For this review, take the finished solid that the model builds, in its own axes (mm). Give positions to 0.01 mm unless a question says otherwise; leave off trailing zeros. Order: outer loops, then holes, each group sorted by start corner. A loop starts at its lowest first (then second) coordinate and runs counter-clockwise, first axis right, second up.
Item 1: For probe 1 along X at (y, z) = (0.3, 96); probe 2 along Y at (x, z) = (0.2, 120); probe 3 along Y at (x, z) = (-0.4, 152), list the stretches that pass through material, from the lowest coordinate up.
Item 2: Consider section A-A (z = 177.5). Give the boundary of the cut face in (x, y).
Item 3: For P1, Ø2, axis at x = -0.5, z = 110, coming from the +Y side; P2, Ø1, axis at x = 1.5, y = 4, coming from the +Z side; P3, Ø1.5, axis at y = 1.5, z = 239.5, coming from the +X side, all flat-tipped, find the tip position at first contact; note any pin that passes through.
Autodesk Inventor part; units mm, degrees
ref_plane "YZ Plane" through (0, 0, 0) normal (1, 0, 0) x (0, 1, 0)
ref_plane "XZ Plane" through (0, 0, 0) normal (0, 1, 0) x (-1, 0, 0)
ref_plane "XY Plane" through (0, 0, 0) normal (0, 0, 1) x (1, 0, 0)
sketch "Szkic1" plane through (0, 0, 0) normal (0, 0, 1) x (1, 0, 0)
  circle A0 centre (0, 0) radius 1
  dimension "d0" = 2
sketch "Szkic4" plane through (0, 0, 0) normal (1, 0, 0) x (0, 1, 0)
  line L0 (0, 0) -> (0, 263.8767)
  arc A0 (1.817, 265.8683) -> (0, 263.8767) centre (2, 263.8767) ccw
  line L1 (1.817, 265.8683) -> (3.25, 266)
  dimension "d2" = 266
  dimension "d3" = 2
  dimension "d4" = 3.25
  dimension "d5" = 95.25
sweep "Szprycha" add profiles "Szkic1" path "Szkic4"
sketch "Szkic5" plane through (0, 0, 0) normal (1, 0, 0) x (0, 1, 0)
  line L0 (3.3415, 265.0042) -> (3.1585, 266.9958) construction
  line L1 (3.1585, 266.9958) -> (3.25, 266)
  line L2 (3.1585, 266.9958) -> (4.1585, 268.1378)
  arc A0 (4.75, 266.1378) -> (4.1585, 268.1378) centre (-0.5843, 265.6477) ccw
  line L3 (1.7255, 266.8641) -> (3.1585, 266.9958) construction
  line L4 (1.9085, 264.8725) -> (3.3415, 265.0042) construction
  line L5 (1.9085, 264.8725) -> (1.7255, 266.8641) construction
  line L6 (1.817, 265.8683) -> (3.25, 266) construction
  line L7 (3.25, 266) -> (4.75, 266.1378)
  point P0 (0, 0)
  dimension "d7" = 1
  dimension "d8" = 1.5
  dimension "d10" = 2
revolve "Główka" add sketch "Szkic5" angle 360 about axis through (0, 3.25, 266) along (0, 0.9958049, 0.0915016)
sketch "Szkic6" plane through (0, 0, 0) normal (0, 0, 1) x (1, 0, 0)
  circle A0 centre (0, 0) radius 1.125
  dimension "d13" = 2.25
extrude "Połączenie z nyplem" add sketch "Szkic6" against normal blind 10.3
chamfer "Faza1" distance 0.2 angle 45 1 edges at (-1.125, 0, -10.3)
thread "Gwint2"
properties part number "Szprycha" material "Aluminium AW-7020"
Resolved:
1. probe 1: x = -0.95 to 0.95
1. probe 2: y = -0.98 to 0.98
1. probe 3: y = -0.92 to 0.92
2. outline: circle Ø2 at (0, 0)
3. P1: stops at y = 1
3. P2: stops at z = 267.86
3. P3: stops at x = 0.66
